Can you work these out from the model? Positions are in its coordinate system, mm. A direction names the side the tool comes from. Round coordinates to 2 decimals unless told otherwise and drop trailing zeros. Order: outer loops, then holes, each group sorted by start corner. A loop starts at its lowest first (then second) coordinate and runs counter-clockwise, first axis right, second up.
Q1. For faces 1 (the face through (3.715, 1.239, 11.549)), 2 (the face through (0, 1.54, 11)), 3 (the face through (0.056, 3.492, 1.127)), 4 (the face through (-3.7, 1.05, 30.21)), which set-ups out of +Z, -Z, +X, -X, +Y, -Y let a thin tool reach every point of the face, with its end or its side?
Q2. Will this pin go through, and if not, where does the flat tip stop? P1, Ø2, axis at x = 1, z = 25.5, coming from the +Y side.
Q3. If we section it at C-C (y = 3.5): Please give me the cut outline in (x, z).
Q4. If we section it at A-A (z = 14): Please give me the cut outline in (x, y), plus the area to 3 significant figures.
Q5. If we section it at B-B (x = -2.5): Please give me the cut outline in (y, z).
Q6. If we section it at D-D (x = 3.5): Please give me the cut outline in (y, z), plus the area to 3 significant figures.
Q7. If I drill on line 1 (Z direction, x = -2.5, y = 3.5); line 2 (Y direction, x = 2.25, z = 16); line 3 (Y direction, x = 0.5, z = 39), over which ranges is the centre line in solid material (lowest first)?
from build123d import *

# Parameters (mm, degrees)
SKETCH1_W               = 8
SKETCH1_H               = 11
BOSS_EXTRUDE1_DEPTH     = 8
SKETCH2_W               = 8
SKETCH2_H               = 7.04
BOSS_EXTRUDE2_DEPTH     = 7
BOSS_EXTRUDE3_DEPTH     = 4
CUT_EXTRUDE_THIN1_DEPTH = 4
FILLET1_R               = 1


with BuildPart() as part:
    # Sketch1 → Boss-Extrude1 (new body)
    with BuildSketch(Plane.XY):
        Rectangle(SKETCH1_W, SKETCH1_H)
    extrude(amount=BOSS_EXTRUDE1_DEPTH)

    # Sketch2 → Boss-Extrude2 (add)
    with BuildSketch(Plane.XY.offset(8)):
        with Locations((0, -1.98)):
            Rectangle(SKETCH2_W, SKETCH2_H)
    extrude(amount=BOSS_EXTRUDE2_DEPTH)

    # Sketch3 → Boss-Extrude3 (add, symmetric)
    with BuildSketch(Plane(origin=(0, 0, 0), x_dir=(0, 0, -1), z_dir=(1, 0, 0))):
        Polygon((-15, 1.54), (-15, -5.5), (-45, -5.5), (-45, 1.14), align=None)
    extrude(amount=BOSS_EXTRUDE3_DEPTH, both=True)

    # Sketch4 → Cut-Extrude-Thin1 (cut, symmetric)
    with BuildSketch(Plane(origin=(0, 0, 0), x_dir=(0, 0, -1), z_dir=(1, 0, 0))):
        Polygon((0, 1.54), (-2.286307066, 5.5), (6.373946972, 10.5), (8.660254038, 6.54), align=None)
    extrude(amount=CUT_EXTRUDE_THIN1_DEPTH, both=True, mode=Mode.SUBTRACT)

    # Fillet1
    fillet1_edges = [part.edges().sort_by_distance(p)[0] for p in [
        (4, 1.54, 11.5),
        (-4, 1.54, 11.5),
        (-4, 1.34, 30),
        (4, 1.34, 30),
        (4, -5.5, 22.5),
        (-4, -5.5, 22.5),
        (0, 5.5, 8),
    ]]
    fillet(fillet1_edges, radius=FILLET1_R)


solid = part.part
Solution:
1. face 1: +Z, +X, +Y
1. face 2: +Z, +X, -X, +Y
1. face 3: -Z, +X, -X, +Y
1. face 4: +Z, -X, +Y
2. P1: stops at y = 1.41
3. outline: (-4, 1.13) - (4, 1.13) - (4, 8) - (-4, 8) - close
4. outline: (-4, -4.5) arc R1 ccw to (-3, -5.5) - (3, -5.5) arc R1 ccw to (4, -4.5) - (4, 0.54) arc R1 ccw to (3, 1.54) - (-3, 1.54) arc R1 ccw to (-4, 0.54) - close
4. area: 55.5 mm2
5. outline: (-5.5, 0) - (1.54, 0) - (5.5, 2.29) - (5.5, 7) arc R1 ccw to (4.5, 8) - (1.54, 8) - (1.54, 15) - (1.14, 45) - (-5.5, 45) - close
6. outline: (-5.37, 0) - (1.54, 0) - (5.5, 2.29) - (5.5, 7) arc R1 ccw to (4.5, 8) - (1.41, 8) - (1.41, 15) - (1.01, 45) - (-5.37, 45) - close
6. area: 327 mm2
7. line 1: z = 1.13 to 8
7. line 2: y = -5.5 to 1.53
7. line 3: y = -5.5 to 1.22
